```python
from build123d import *

# Parameters (mm, degrees)
EXTRUDE_14_DEPTH     = 34
SKETCH_41_R          = 2.75
CUT_EXTRUDE_27_DEPTH = 86.772956111
SKETCH_42_R          = 2.75
CUT_EXTRUDE_28_DEPTH = 86.772956111


with BuildPart() as part:
    # Sketch 40 → Extrude 14 (new body)
    with BuildSketch(Plane.XY):
        with BuildLine():
            Line((40, 9), (9, 40))
            Line((9, 40), (9, 59))
            ThreePointArc((9, 59), (8.707106781, 59.707106781), (8, 60))
            Line((8, 60), (1, 60))
            ThreePointArc((1, 60), (0.292893219, 59.707106781), (0, 59))
            Line((0, 59), (0, 1))
            ThreePointArc((0, 1), (0.292893219, 0.292893219), (1, 0))
            Line((1, 0), (59, 0))
            ThreePointArc((59, 0), (59.707106781, 0.292893219), (60, 1))
            Line((60, 1), (60, 8))
            ThreePointArc((60, 8), (59.707106781, 8.707106781), (59, 9))
            Line((59, 9), (40, 9))
        make_face()
        with BuildLine():
            Line((6, 12), (7.428034206, 12))
            ThreePointArc((7.428034206, 12), (7.761575809, 12.12750839), (7.925, 12.445000003))
            ThreePointArc((7.925, 12.445000003), (9.455281371, 15.213766145), (12.501000018, 16.068999998))
            ThreePointArc((12.501000018, 16.068999998), (12.854580587, 15.852403207), (12.923122843, 15.443459021))
            Line((12.923122843, 15.443459021), (12.661152875, 14.464571239))
            ThreePointArc((12.661152875, 14.464571239), (12.468861172, 14.18703128), (12.144000016, 14.094999999))
            ThreePointArc((12.144000016, 14.094999999), (10.51595825, 10.514958251), (14.095999999, 12.143000014))
            ThreePointArc((14.095999999, 12.143000014), (14.18803128, 12.467861171), (14.465571239, 12.660152875))
            Line((14.465571239, 12.660152875), (15.444578727, 12.922154879))
            ThreePointArc((15.444578727, 12.922154879), (15.853118545, 12.853885203), (16.07, 12.501))
            ThreePointArc((16.07, 12.501), (15.215158242, 9.454636451), (12.446000002, 7.924))
            ThreePointArc((12.446000002, 7.924), (12.127844119, 7.760840711), (12, 7.426924553))
            Line((12, 7.426924553), (12, 5.5))
            ThreePointArc((12, 5.5), (12.146446609, 5.146446609), (12.5, 5))
            Line((12.5, 5), (37.844, 5))
            ThreePointArc((37.844, 5), (38.305045436, 5.30916781), (38.196447939, 5.853552061))
            Line((38.196447939, 5.853552061), (5.853553317, 38.196446683))
            ThreePointArc((5.853553317, 38.196446683), (5.308658302, 38.304832993), (5, 37.842893363))
            Line((5, 37.842893363), (5, 13))
            ThreePointArc((5, 13), (5.292893219, 12.292893219), (6, 12))
        make_face(mode=Mode.SUBTRACT)
    extrude(amount=-EXTRUDE_14_DEPTH)

    # Sketch 41 → Cut-Extrude 27 (cut, through all)
    with BuildSketch(Plane(origin=(0, 9, 0), x_dir=(1, 0, 0), z_dir=(0, 1, 0))):
        with Locations(Location((50, 27, 0), (0, 0, 270))):
            Circle(SKETCH_41_R)
        with Locations(Location((50, 7, 0), (0, 0, 270))):
            Circle(SKETCH_41_R)
    extrude(amount=-CUT_EXTRUDE_27_DEPTH, mode=Mode.SUBTRACT)

    # Sketch 42 → Cut-Extrude 28 (cut, through all)
    with BuildSketch(Plane(origin=(9, 0, 0), x_dir=(0, 0, -1), z_dir=(1, 0, 0))):
        with Locations(Location((7, 50, 0), (0, 0, 90))):
            Circle(SKETCH_42_R)
        with Locations(Location((27, 50, 0), (0, 0, 90))):
            Circle(SKETCH_42_R)
    extrude(amount=-CUT_EXTRUDE_28_DEPTH, mode=Mode.SUBTRACT)


solid = part.part
```
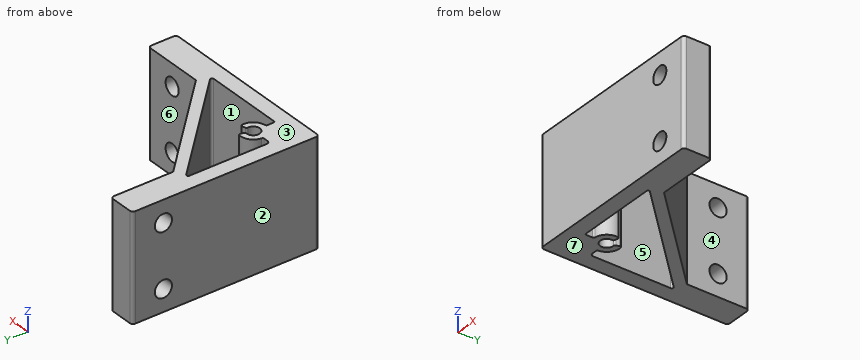
Source: CAD feature listing. Evaluate the final solid. Frame: model axes, mm. Face numbers are marked on the shaded views. A direction names the side the tool comes from. Give positions to 0.01 mm unless a question says otherwise; leave off trailing zeros. Order: outer loops, then holes, each group sorted by start corner. A loop starts at its lowest first (then second) coordinate and runs counter-clockwise, first axis right, second up.
(1) Material intervals for line 1 along Z through (x, y) = (6, 50); line 2 along Y through (x, z) = (11, -6.5); line 3 along Y through (x, z) = (43, -8), sorted ascending.
(2) Pull-direction query (X, two-part tool) for the marked faces 1, 2, 3 and 4; classes: +X half, -X half, draft (parallel to the pull), parting line (faces both ways), or undercut.
(3) Access query for the marked faces 5, 6 and 7. Directions: +Z, -Z, +X, -X, +Y, -Y. A direction counts if a zero-diameter tool reaches every point of the face in a straight line with its end or side. Return the directions, or none.
(4) Section query B-B (x = 32). Return the cut outline in (y, z), plus the area to 3 significant figures.
(5) Section query A-A (y = 26). Return the cut outline in (x, z).
(6) Section query C-C (x = 50). Return the cut outline in (y, z), plus the area to 3 significant figures.
(7) Section query D-D (z = -25). State how many separate pieces and enclosed holes the cut face has, plus the area to 3 significant figures.
(8) Contact query for flat-ended pins moving along their axis: P1, Ø5, axis at y = 50, z = -27, coming from the -X side; P2, Ø1, axis at x = 20.5, z = -21.5, coming from the -Y side; P3, Ø12.5, axis at y = 25, z = -10.5, coming from the +X side; P4, Ø5.5, axis at x = 46, z = -18.5, coming from the +Y side. Output: stop coordinate, or through.
Outcome:
1. line 1: z = -34 to -29.75, -24.25 to -9.75, -4.25 to 0
1. line 2: y = 0 to 10.15, 13.85 to 15.98, 33.05 to 38
1. line 3: y = 0 to 9
2. face 1: undercut
2. face 2: -X half
2. face 3: draft
2. face 4: +X half
3. face 5: +Z, -Z
3. face 6: +Z, -Z, +X, +Y
3. face 7: -Z, +X, -X, +Y, -Y
4. outline: (0, -34) - (5, -34) - (5, 0) - (0, 0) - close; (12.05, -34) - (17, -34) - (17, 0) - (12.05, 0) - close
4. area: 338 mm2
5. outline: (0, -34) - (5, -34) - (5, 0) - (0, 0) - close; (18.05, -34) - (23, -34) - (23, 0) - (18.05, 0) - close
6. outline: (0, -34) - (9, -34) - (9, -29.75) - (0, -29.75) - close; (0, -24.25) - (9, -24.25) - (9, -9.75) - (0, -9.75) - close; (0, -4.25) - (9, -4.25) - (9, 0) - (0, 0) - close
6. area: 207 mm2
7. separate pieces: 3
7. enclosed holes: 1
7. area: 900 mm2
8. P1: passes through
8. P2: stops at y = 0
8. P3: stops at x = 30.25
8. P4: stops at y = 9
